Input: part model. Units: mm. Frame: model coordinates. Give positions to 0.01 mm unless a question says otherwise; leave off trailing zeros. Loops run counter-clockwise (first coordinate to the right, second up) from the corner with the lowest first, then second, coordinate; pieces in that order, holes last.
from build123d import *

# Parameters (mm, degrees)
SKETCH1_W           = 15
SKETCH1_H           = 15
BOSS_EXTRUDE1_DEPTH = 785
SKETCH2_R           = 3
CUT_EXTRUDE1_DEPTH  = 5
CUT_EXTRUDE2_START  = -5
SKETCH3_R           = 3
CUT_EXTRUDE2_DEPTH  = 5
FILLET1_R           = 1
SKETCH5_R           = 3
CUT_EXTRUDE4_DEPTH  = 786.286571896


with BuildPart() as part:
    # Sketch1 → Boss-Extrude1 (new body)
    with BuildSketch(Plane.XY):
        with Locations((7.5, 7.5)):
            Rectangle(SKETCH1_W, SKETCH1_H)
    extrude(amount=BOSS_EXTRUDE1_DEPTH)

    # Sketch2 → Cut-Extrude1 (cut)
    with BuildSketch(Plane(origin=(0, 0, 0), x_dir=(-1, 0, 0), z_dir=(0, 0, -1))):
        with Locations((-7.5, 7.5)):
            Circle(SKETCH2_R)
    extrude(amount=-CUT_EXTRUDE1_DEPTH, mode=Mode.SUBTRACT)

    # Sketch3 → Cut-Extrude2 (cut)
    with BuildSketch(Plane.XY.offset(785).offset(CUT_EXTRUDE2_START)):
        with Locations(Location((7.5, 7.5, 0), (0, 0, 180))):
            Circle(SKETCH3_R)
    extrude(amount=CUT_EXTRUDE2_DEPTH, mode=Mode.SUBTRACT)

    # Fillet1
    fillet1_edges = [part.edges().sort_by_distance(p)[0] for p in [
        (0, 7.5, 785),
        (7.5, 0, 785),
        (15, 7.5, 785),
        (7.5, 0, 0),
        (0, 7.5, 0),
        (7.5, 15, 0),
        (15, 7.5, 0),
        (15, 0, 392.5),
        (0, 0, 392.5),
        (0, 15, 392.5),
        (15, 15, 392.5),
        (7.5, 15, 785),
    ]]
    fillet(fillet1_edges, radius=FILLET1_R)

    # Sketch5 → Cut-Extrude4 (cut, through all)
    with BuildSketch(Plane(origin=(15, 0, 0), x_dir=(0, 0, -1), z_dir=(1, 0, 0))):
        with Locations((-101, 7.5)):
            Circle(SKETCH5_R)
        with Locations((-634, 7.5)):
            Circle(SKETCH5_R)
    extrude(amount=-CUT_EXTRUDE4_DEPTH, mode=Mode.SUBTRACT)


solid = part.part
(1) Pin query (flat end, axial travel): pin 1 Ø1.8 at (x, y) = (7.5, 6) entering from +Z; pin 2 Ø3 at (x, y) = (6.5, 7) entering from -Z. Return the tip coordinate at first contact, or that it passes through.
Values follow:
pin 1: stops at z = 780
pin 2: stops at z = 5
(2) Cut plane A-A (y = 7.5). Return the cut outline in (x, z).
Values follow:
outline: (0, 1) arc R1 ccw to (1, 0) - (4.5, 0) - (4.5, 5) - (10.5, 5) - (10.5, 0) - (14, 0) arc R1 ccw to (15, 1) - (15, 98) - (0, 98) - close; (0, 104) - (15, 104) - (15, 631) - (0, 631) - close; (0, 637) - (15, 637) - (15, 784) arc R1 ccw to (14, 785) - (10.5, 785) - (10.5, 780) - (4.5, 780) - (4.5, 785) - (1, 785) arc R1 ccw to (0, 784) - close
(3) Ray query, probe 1 along Z at (x, y) = (8.5, 7.25); probe 2 along X at (y, z) = (7.5, 781.9); probe 3 along Z at (x, y) = (8, 5.5). Return the intervals inside material, ascending.
Values follow:
probe 1: z = 5 to 98.01, 103.99 to 631.01, 636.99 to 780
probe 2: x = 0 to 4.5, 10.5 to 15
probe 3: z = 5 to 98.76, 103.24 to 631.76, 636.24 to 780
